Input: part model. Units: mm. Frame: model coordinates. A direction names the side the tool comes from. Round coordinates to 2 decimals unless told otherwise and drop trailing zeros. Write each loop counter-clockwise with the first axis right and the second up, starting at its lowest first coordinate (ties: lowest second). Pieces come first, ordered by that corner, then holes. Notation, with made-up numbers: M 63,-26.75 L 84,-26.75 A11 cw 84,-7.75 Z; hole C -20,-28 d4. An arc over 180 degrees is marked long. Answer as CSV lines item,"result". Start each with the question number.
```python
from build123d import *

# Parameters (mm, degrees)
BOSS_EXTRU_1_DEPTH      = 8
ESQUISSE2_R             = 2.45
ENL_V_MAT_EXTRU_1_DEPTH = 4
ENL_V_MAT_EXTRU_2_REACH = 6
ESQUISSE3_R             = 1.75
ESQUISSE4_R             = 3.75
ENL_V_MAT_EXTRU_3_DEPTH = 2.5
ENL_V_MAT_EXTRU_4_DEPTH = 4
CHANFREIN1_SIZE         = 1


with BuildPart() as part:
    # Esquisse1 → Boss.-Extru.1 (new body)
    with BuildSketch(Plane(origin=(0, 0, 0), x_dir=(1, 0, 0), z_dir=(0, 1, 0))):
        with BuildLine():
            Line((-3, 26.381049961), (-3, 4.963869458))
            ThreePointArc((-3, 4.963869458), (0, -5.8), (3, 4.963869458))
            Line((3, 4.963869458), (3, 38.463869458))
            Line((3, 38.463869458), (-0.867157449, 56.657414832))
            Line((-0.867157449, 56.657414832), (-1.84530505, 56.449503141))
            ThreePointArc((-1.84530505, 56.449503141), (-3.756758837, 55.119060789), (-4.140414176, 52.821988519))
            Line((-4.140414176, 52.821988519), (-3, 49.618950039))
            ThreePointArc((-3, 49.618950039), (0, 38), (-3, 26.381049961))
        make_face()
    extrude(amount=BOSS_EXTRU_1_DEPTH)

    # Esquisse2 → Enlèv. mat.-Extru.1 (cut)
    with BuildSketch(Plane(origin=(0, 8, 0), x_dir=(1, 0, 0), z_dir=(0, 1, 0))):
        Circle(ESQUISSE2_R)
    extrude(amount=-ENL_V_MAT_EXTRU_1_DEPTH, mode=Mode.SUBTRACT)

    # Esquisse3 → Enlèv. mat.-Extru.2 (cut, up to next)
    with BuildSketch(Plane(origin=(0, 4, 0), x_dir=(1, 0, 0), z_dir=(0, 1, 0)), mode=Mode.PRIVATE) as enl_v_mat_extru_2_sk1:
        Circle(ESQUISSE3_R)
    enl_v_mat_extru_2_tool1 = extrude(enl_v_mat_extru_2_sk1.sketch, amount=-ENL_V_MAT_EXTRU_2_REACH, mode=Mode.PRIVATE) & part.part
    add(enl_v_mat_extru_2_tool1.solids().sort_by_distance((0, 4, 0))[0], mode=Mode.SUBTRACT)

    # Esquisse4 → Enlèv. mat.-Extru.3 (cut)
    with BuildSketch(Plane.XZ):
        Circle(ESQUISSE4_R)
    extrude(amount=-ENL_V_MAT_EXTRU_3_DEPTH, mode=Mode.SUBTRACT)

    # Esquisse5 → Enlèv. mat.-Extru.4 (cut)
    with BuildSketch(Plane(origin=(0, 8, 0), x_dir=(1, 0, 0), z_dir=(0, 1, 0))):
        with BuildLine():
            Line((-3, 4.963869458), (-3, 17.24093965))
            ThreePointArc((-3, 17.24093965), (0, 17.5), (3, 17.24093965))
            Line((3, 17.24093965), (3, 4.963869458))
            ThreePointArc((3, 4.963869458), (0, 5.8), (-3, 4.963869458))
        make_face()
    extrude(amount=-ENL_V_MAT_EXTRU_4_DEPTH, mode=Mode.SUBTRACT)

    # Chanfrein1
    chanfrein1_edges = [part.edges().sort_by_distance(p)[0] for p in [
        (-2.45, 8, 0),
    ]]
    chamfer(chanfrein1_edges, length=CHANFREIN1_SIZE)


solid = part.part
```
Item 1: Cut plane B-B, the plane z = -9. Return loops of the section in (x, y).
Item 2: Cut plane A-A, the plane z = 0. Return loops of the section in (x, y), plus the area to 3 significant figures.
Item 3: Draft query along X for faces 1 (the face through (-1.349, 3.944, -56.555)), 2 (the face through (3, 4, -25)), 3 (the face through (2, 2.5, -1)). Return one class per face: +X half, -X half, draft (parallel to the pull), parting line (faces both ways), or undercut.
Item 4: Pin query (flat end, axial travel): pin 1 Ø4 at (y, z) = (2, -18.5) entering from -X; pin 2 Ø3 at (x, y) = (0.5, 3.5) entering from -Z; pin 3 Ø4 at (x, z) = (1.5, -1) entering from -Y; pin 4 Ø2.5 at (y, z) = (2, -25) entering from +X. Return the tip coordinate at first contact, or that it passes through.
Item 5: Line query: line 1 (X direction, y = 3.55, z = 0); line 2 (X direction, y = 5.7, z = 0); line 3 (Y direction, x = -1.25, z = -7). Output: solid intervals per line, ascending. Write a range as [from, to].
Item 6: Access query for faces 4 (the face through (0.14, 8, -37.23)), 5 (the face through (0, 6, -17.5)), 6 (the face through (0, 0, -19)), 7 (the face through (-3, 3, -18)), 8 (the face through (-3.746, 1.232, 0.165)). Directions: +Z, -Z, +X, -X, +Y, -Y. A direction counts if a zero-diameter tool reaches every point of the face in a straight line with its end or side. Return the directions, or none.
Item 7: Cut plane C-C, the plane x = 5.25. Return loops of the section in (y, z), plus the area to 3 significant figures.
Results list:
1,outline,"M -3,0 L 3,0 L 3,4 L -3,4 Z"
2,outline,"M -5.8,0 L -3.75,0 L -3.75,2.5 L -1.75,2.5 L -1.75,4 L -2.45,4 L -2.45,7 L -3.45,8 L -5.8,8 Z; M 1.75,2.5 L 3.75,2.5 L 3.75,0 L 5.8,0 L 5.8,8 L 3.45,8 L 2.45,7 L 2.45,4 L 1.75,4 Z"
2,area,"48.2 mm²"
3,face 1,"-X half"
3,face 2,"+X half"
3,face 3,"undercut"
4,pin 1,"x = -3"
4,pin 2,"z = -56.66"
4,pin 3,"y = 0"
4,pin 4,"x = 3"
5,line 1,"[-5.8, -1.75], [1.75, 5.8]"
5,line 2,"[-5.8, -2.45], [2.45, 5.8]"
5,line 3,"[0, 4]"
6,face 4,"+Z, -Z, +X, -X, +Y"
6,face 5,"+Y"
6,face 6,"+Z, -Z, +X, -X, -Y"
6,face 7,"-X, +Y, -Y"
6,face 8,"-Y"
7,outline,"M 0,-2.47 L 8,-2.47 L 8,2.47 L 0,2.47 Z"
7,area,"39.4 mm²"
